The model under review builds one solid part; all positions refer to its coordinate system, in mm. A direction names the side the tool comes from. Give positions to 0.01 mm unless a question says otherwise; leave off trailing zeros. Order: outer loops, then holes, each group sorted by start corner. A loop starts at its lowest first (then second) coordinate and runs counter-clockwise, first axis right, second up. Notation, with made-up numbers: (-31, 2.5) -> (15, 2.5) arc R28 ccw to (15, 26.5) -> close; hole circle Ø5 at (40, 55). An arc over 180 degrees is marked (long way). Answer as a JSON object with one key per item and string values. Group by question number.
Autodesk Fusion 360 part; units mm, degrees
sketch "Front" plane through (0, 0, 0) normal (0, 1, 0) x (1, 0, 0)
  line L0 (-75, -10) -> (75, -10) construction
  line L1 (-75, -24) -> (75, -24) construction
  line L2 (-75, -74.5651) -> (75, -74.5651) construction
  line L3 (-74, -51.5) -> (76, -51.5) construction
  circle A0 centre (1, -51.5) radius 32.5
  circle A1 centre (1, -51.5) radius 41.5
  line L4 (-48.5, 10) -> (-48.5, -85) construction
  line L5 (50.5, 10) -> (50.5, -85) construction
  line L6 (65, 10) -> (65, -25) construction
  line L7 (-63, 10) -> (-63, -25) construction
  line L8 (-33.5, -74.5651) -> (-48.5, -74.5651)
  line L9 (-48.5, -74.5651) -> (-48.5, -24)
  line L10 (-48.5, -24) -> (-63, -24)
  line L11 (-63, -24) -> (-63, -10)
  line L12 (-63, -10) -> (65, -10)
  line L13 (65, -10) -> (65, -24)
  line L14 (65, -24) -> (50.5, -24)
  line L15 (50.5, -24) -> (50.5, -74.5651)
  line L16 (50.5, -74.5651) -> (35.5, -74.5651)
  line L17 (-30, -53) -> (-51, -53)
  line L18 (-51, -53) -> (-51, -50)
  line L19 (-51, -50) -> (-30, -50)
  line L20 (-30, -50) -> (-30, -53)
  line L21 (-30, -53) -> (-51, -50) construction
  line L22 (-51, -53) -> (-30, -50) construction
  point P0 (-33.5, -74.5651)
  point P1 (35.5, -74.5651)
  point P2 (0.9773, -10)
  point P3 (-40.5, -51.5)
  dimension "d1" = 14
  dimension "d2" = 65
  dimension "d3" = 83
  dimension "d4" = 49.5
  dimension "d5" = 49.5
  dimension "d6" = 64
  dimension "d7" = 64
  dimension "d8" = 15
  dimension "d9" = 15
  dimension "d10" = 23.0651
  dimension "d14" = 14.5
  dimension "d15" = 3
extrude "Extrude1" add sketch "Front" along normal blind 78 contours A0 A1 L17 L19 | A1 L9 L10 L11 L12 L19 | A1 L8 L9 L17 | A1 L12 L13 L14 L15 L16 picked at (34.7953, -69.7412)
sketch "Top holes" plane through (0, 0, 74.5651) normal (0, 0, 1) x (-1, 0, 0)
  line L0 (48.5, 0) -> (33.5, 0)
  line L1 (33.5, 0) -> (33.5, -78)
  line L2 (33.5, -78) -> (48.5, -78)
  line L3 (48.5, -78) -> (48.5, 0)
  line L4 (41, -78) -> (41, 0) construction
  circle A0 centre (41, -39) radius 7
  circle A1 centre (41, -64) radius 7
  circle A2 centre (41, -14) radius 7
  circle A3 centre (41, -39) radius 4
  circle A4 centre (41, -64) radius 4
  circle A5 centre (41, -14) radius 4
  dimension "d18" = 14
  dimension "d19" = 14
  dimension "d20" = 14
  dimension "d21" = 25
  dimension "d22" = 25
  dimension "d23" = 8
  dimension "d24" = 8
  dimension "d25" = 8
extrude "Extrude2" cut sketch "Top holes" against normal blind 45 contours A4 | A5
extrude "Extrude5" cut sketch "Top holes" against normal blind 23 contours A3
extrude "Extrude3" cut sketch "Top holes" against normal blind 10 contours A0 | A1 | A2
sketch "Bottom holes" plane through (0, 0, 10) normal (0, 0, -1) x (1, 0, 0)
  line L0 (65, 0) -> (-63, 0)
  line L1 (-63, -78) -> (65, -78)
  line L2 (65, -78) -> (65, 0)
  line L3 (1, -78) -> (1, 0) construction
  line L4 (55, -47) -> (-53, -47) construction
  line L5 (-53, -47) -> (-53, -25) construction
  line L6 (-53, -25) -> (55, -25) construction
  line L7 (55, -25) -> (55, -47) construction
  line L8 (55, -47) -> (-53, -25) construction
  line L9 (-53, -47) -> (55, -25) construction
  circle A0 centre (-53, -25) radius 3
  circle A1 centre (-53, -47) radius 3
  circle A2 centre (55, -47) radius 3
  circle A3 centre (55, -25) radius 3
  line L10 (-63, 0) -> (-63, -78)
  point P0 (1, -36)
  dimension "d38" = 108
  dimension "d39" = 22
  dimension "d40" = 25
  dimension "d41" = 6
  dimension "d42" = 6
  dimension "d43" = 6
  dimension "d44" = 6
extrude "Extrude4" cut sketch "Bottom holes" against normal through all contours A0 | A1 | A2 | A3
equation "d3 = d2 + 18 mm"
equation "d4 = ( 99 / 2 ) * 1 mm"
equation "d5 = d4"
equation "d7 = d6"
equation "d19 = d18"
equation "d20 = d18"
equation "d22 = d21"
equation "d24 = d23"
equation "d25 = d23"
equation "d42 = d41"
equation "d43 = d41"
equation "d44 = d41"
1. Machinability: for faces 1 (the flat face through (-44, 42, 64.565)), 2 (the cylindrical face through (52, 25, 17)), 3 (the flat face through (43, 38, 74.565)), 4 (the flat face through (-41, 47, 74.565)), which of the approach directions +Z, -Z, +X, -X, +Y, -Y give a long, thin tool a straight path to every point of the face, cutting with its end or side? Answer none if there is none.
2. For pin 1 (9 mm diameter, centred on x = -41, y = 14, fed in from +Z); pin 2 (1.5 mm diameter, centred on x = 50.5, y = 47.5, fed in from +Z); pin 3 (6.5 mm diameter, centred on x = -41, y = 14, fed in from +Z), all flat-tipped, find the tip position at first contact; note any pin that passes through.
3. Take a section at B-B on y = 64. Give the boundary of the cut face in (x, z), plus the area to 3 significant figures.
4. Take a section at C-C on z = 70.5. Give the boundary of the cut face in (x, y).
5. For probe 1 along Y at (x, z) = (-41, 34.5); probe 2 along Y at (x, z) = (-41, 71.5); probe 3 along X at (y, z) = (47, 15.25), list the stretches that pass through material, from the lowest coordinate up. Write a range as [from, to].
6. Draft analysis for pull direction X (two halves, no side actions). For faces 5 (the flat face through (0, 0, 14)), 6 (the flat face through (-48.5, 38, 37)), 7 (the cylindrical face through (-40.133, 67.905, 58.864)), state which applies: pulls with the +X half, pulls with the -X half, needs draft (parallel to the pull), parting line crosses it, or undercut.
7. Take a section at A-A on z = 32. Give the boundary of the cut face in (x, y), plus the area to 3 significant figures.
8. Take a section at D-D on x = 1. Give the boundary of the cut face in (y, z).
Checks:
{
 "1": {"face 1": "+Z", "face 2": "+Z, -Z", "face 3": "+Z, +X, +Y, -Y", "face 4": "+Z, -X, +Y, -Y"},
 "2": {"pin 1": "stops at z = 64.57", "pin 2": "stops at z = 74.57", "pin 3": "stops at z = 29.57"},
 "3": {"outline": "(-63, 10) -> (65, 10) -> (65, 24) -> (50.5, 24) -> (50.5, 74.57) -> (35.5, 74.57) arc R41.5 ccw to (-33.5, 74.57) -> (-34, 74.57) -> (-34, 64.57) -> (-37, 64.57) -> (-37, 53) -> (-31.47, 53) arc R32.5 cw (long way) to (-31.47, 50) -> (-37, 50) -> (-37, 29.57) -> (-45, 29.57) -> (-45, 50) -> (-48.5, 50) -> (-48.5, 24) -> (-63, 24) -> close; (-48.5, 53) -> (-45, 53) -> (-45, 64.57) -> (-48, 64.57) -> (-48, 74.57) -> (-48.5, 74.57) -> close", "area": "3,930 mm2"},
 "4": {"outline": "(-48.5, 0) -> (-25.37, 0) -> (-25.37, 78) -> (-48.5, 78) -> close; (27.37, 0) -> (50.5, 0) -> (50.5, 78) -> (27.37, 78) -> close; hole circle Ø14 at (-41, 14); hole circle Ø14 at (-41, 39); hole circle Ø14 at (-41, 64)"},
 "5": {"probe 1": "y = [0, 10], [18, 60], [68, 78]", "probe 2": "y = [0, 7], [21, 32], [46, 57], [71, 78]", "probe 3": "x = [-63, -56], [-50, 52], [58, 65]"},
 "6": {"face 5": "needs draft", "face 6": "pulls with the -X half", "face 7": "undercut"},
 "7": {"outline": "(-48.5, 0) -> (-25, 0) -> (-25, 78) -> (-48.5, 78) -> close; (27, 0) -> (50.5, 0) -> (50.5, 78) -> (27, 78) -> close; hole circle Ø8 at (-41, 14); hole circle Ø8 at (-41, 64)", "area": "3,570 mm2"},
 "8": {"outline": "(0, 10) -> (78, 10) -> (78, 19) -> (0, 19) -> close; (0, 84) -> (78, 84) -> (78, 93) -> (0, 93) -> close"}
}
